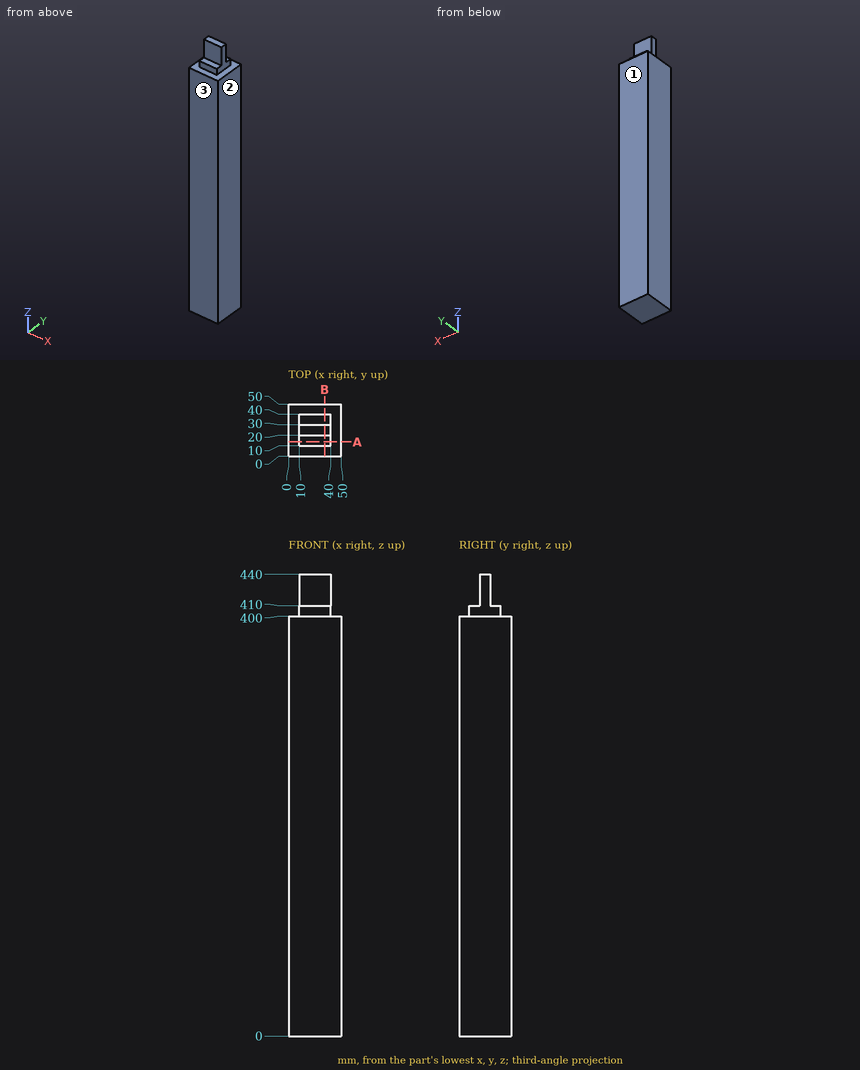
Could you check a few things on this drawing? It's one solid part, dimensions in mm from its lowest x, y, z. Round coordinates to 2 decimals unless told otherwise and drop trailing zeros. Order: outer loops, then holes, each group sorted by start corner. A loop starts at its lowest first (then second) coordinate and runs counter-clockwise, first axis right, second up. Notation, with made-up numbers: M 18,-27.5 L 29,-27.5 A23 ccw 29,0.5 Z; hole C 62.25,56 d4. An arc over 180 degrees is marked long. Use a Markdown table: item, result.
1) Imagine slicing it at A-A (y = 14). List the corners of the cut face in (x, z) for me, then the cut area to 3 significant figures.
Geometry says:
| item | result |
|---|---|
| outline | M 0,0 L 50,0 L 50,400 L 40,400 L 40,410 L 10,410 L 10,400 L 0,400 Z |
| area | 20,300 mm² |
2) If we mould it in two halves opening along Y, with no side actions, what happens to the marked faces 1, 2 and 3? For each: +Y half, -Y half, draft (parallel to the pull), parting line (faces both ways), or undercut.
Geometry says:
| item | result |
|---|---|
| face 1 | +Y half |
| face 2 | draft |
| face 3 | -Y half |
3) Imagine slicing it at B-B (x = 34.5). List the corners of the cut face in (y, z) for me.
Geometry says:
| item | result |
|---|---|
| outline | M 0,0 L 50,0 L 50,400 L 40,400 L 40,410 L 30,410 L 30,440 L 20,440 L 20,410 L 10,410 L 10,400 L 0,400 Z |
4) I'm going to push flat-ended pins straight in: P1, Ø3, axis at x = 32.5, z = 405.5, coming from the -Y side; P2, Ø12, axis at x = 10, y = 9.5, coming from the -Z side; P3, Ø3, axis at x = 27.5, z = 407.5, coming from the +Y side; P4, Ø24, axis at y = 25.5, z = 421, coming from the +X side. Where does each tip first touch, or does it pass through?
Geometry says:
| item | result |
|---|---|
| P1 | stops at y = 10 |
| P2 | stops at z = 0 |
| P3 | stops at y = 40 |
| P4 | stops at x = 40 |
5) If I drill on line 1 along Z through (x, y) = (41.5, 27); line 2 along Z through (x, y) = (22, 38.5), over which ranges is the centre line in solid material (lowest first)?
Geometry says:
| item | result |
|---|---|
| line 1 | z = 0 to 400 |
| line 2 | z = 0 to 410 |
